from build123d import *

# Parameters (mm, degrees)
BOSS_EXTRUDE1_DEPTH      = 15
BOSS_EXTRUDE1_DEPTH_BACK = 15
SKETCH3_R                = 2.5
CUT_EXTRUDE1_DEPTH       = 15


with BuildPart() as part:
    # Sketch2 → Boss-Extrude1 (new, two sides: drawn at the far end of the back side and taken through both)
    with BuildSketch(Plane.XY.offset(-BOSS_EXTRUDE1_DEPTH_BACK)):
        Polygon((-60.5, 0), (-60.5, 27), (0, 27), (0, 37), (-70.5, 37), (-70.5, 10), (-85.5, 10), (-85.5, 0), align=None)
    extrude(amount=BOSS_EXTRUDE1_DEPTH + BOSS_EXTRUDE1_DEPTH_BACK)

    # Mirror1: part across plane


with BuildPart() as part_1:
    add(part.part)
    add(part.part.mirror(Plane(origin=(0, 0, 0), x_dir=(0, 0, 1), z_dir=(1, 0, 0))))

    # Sketch3 → Cut-Extrude1 (cut)
    with BuildSketch(Plane(origin=(0, 10, 0), x_dir=(1, 0, 0), z_dir=(0, 1, 0))):
        with Locations(Location((-78, 0, 0), (0, 0, 270))):
            Circle(SKETCH3_R)
        with Locations(Location((78, 0, 0), (0, 0, 90))):
            Circle(SKETCH3_R)
    extrude(amount=-CUT_EXTRUDE1_DEPTH, mode=Mode.SUBTRACT)


solid = part_1.part
CAD build for the part. Positions are in the model's coordinates, mm. A direction names the side the tool comes from. Round coordinates to 2 decimals unless told otherwise and drop trailing zeros. Write each loop counter-clockwise with the first axis right and the second up, starting at its lowest first coordinate (ties: lowest second). Pieces come first, ordered by that corner, then holes. Notation, with made-up numbers: M 65.25,25 L 80.25,25 A22 cw 80.25,47 Z; hole C 53.25,-20 d7. An arc over 180 degrees is marked long. Put each result on its own line as item: value. Start each with the question number.
1) Drill centre lines: probe 1 along X at (y, z) = (5.25, 0); probe 2 along Z at (x, y) = (78, 4.75); probe 3 along X at (y, z) = (25, 5.25). Where is each one in solid material? Low to high. Write a range as [from, to].
2) Saw through at C-C, the plane x = 78. Write the cut outline in (y, z).
3) Pin check, flat tips, straight feed: pin 1 Ø7.5 at (x, z) = (79.5, 4.5) entering from +Y; pin 2 Ø13.5 at (y, z) = (17.5, 2) entering from -X; pin 3 Ø8 at (y, z) = (18, -6.5) entering from +X. Stop position of each tip, or through.
4) Saw through at A-A, the plane z = 0. Write the cut outline in (x, y).
5) Saw through at D-D, the plane z = -6.25. Write the cut outline in (x, y).
6) Pull direction Z, two halves, no side cores. Call faces 6 (the flat face through (81, 10, 0)), 7 (the cylindrical face through (80.22, 5.07, -1.15)), 8 (the flat face through (0, 30, 15)): pulls with the +Z half, pulls with the -Z half, needs draft (parallel to the pull), parting line crosses it, or undercut.
7) Saw through at B-B, the plane y = 4. Write the cut outline in (x, z), and give its area (3 significant figures).
8) 3-axis set-ups, long thin cutter, end or side, ignore diameter. For faces 1 (the cylindrical face through (-80.22, 5.07, 1.15)), 2 (the flat face through (60.5, 13, 0)), 3 (the flat face through (-85.5, 5, 0)), 4 (the flat face through (-70.5, 24, 0)), 5 (the flat face through (70.5, 24, 0)): which of +Z, -Z, +X, -X, +Y, -Y reach the whole face in a straight line?
Resolved:
1. probe 1: [-85.5, -80.5], [-75.5, -60.5], [60.5, 75.5], [80.5, 85.5]
1. probe 2: [-15, -2.5], [2.5, 15]
1. probe 3: [-70.5, -60.5], [60.5, 70.5]
2. outline: M 0,-15 L 10,-15 L 10,-2.5 L 0,-2.5 Z; M 0,2.5 L 10,2.5 L 10,15 L 0,15 Z
3. pin 1: y = 10
3. pin 2: x = -70.5
3. pin 3: x = 70.5
4. outline: M -85.5,0 L -80.5,0 L -80.5,10 L -85.5,10 Z; M -75.5,0 L -60.5,0 L -60.5,27 L 60.5,27 L 60.5,0 L 75.5,0 L 75.5,10 L 70.5,10 L 70.5,37 L -70.5,37 L -70.5,10 L -75.5,10 Z; M 80.5,0 L 85.5,0 L 85.5,10 L 80.5,10 Z
5. outline: M -85.5,0 L -60.5,0 L -60.5,27 L 60.5,27 L 60.5,0 L 85.5,0 L 85.5,10 L 70.5,10 L 70.5,37 L -70.5,37 L -70.5,10 L -85.5,10 Z
6. face 6: needs draft
6. face 7: undercut
6. face 8: pulls with the +Z half
7. outline: M -85.5,-15 L -60.5,-15 L -60.5,15 L -85.5,15 Z; M 60.5,-15 L 85.5,-15 L 85.5,15 L 60.5,15 Z; hole C -78,0 d5; hole C 78,0 d5
7. area: 1,460 mm²
8. face 1: +Y, -Y
8. face 2: +Z, -Z, -Y
8. face 3: +Z, -Z, -X, +Y, -Y
8. face 4: +Z, -Z, -X, +Y
8. face 5: +Z, -Z, +X, +Y
